Verification items for the finished model (mm, model axes). Coordinates: 2 decimals unless noted, no trailing zeros. Write each loop counter-clockwise with the first axis right and the second up, starting at its lowest first coordinate (ties: lowest second). Pieces come first, ordered by that corner, then holes. Notation, with made-up numbers: (53.5, 11.5) -> (101.5, 11.5) arc R23 ccw to (101.5, 33.5) -> close; hole circle Ø4 at (50.25, 81). An arc over 180 degrees is marked (long way). Answer in a Markdown table with one row per item.
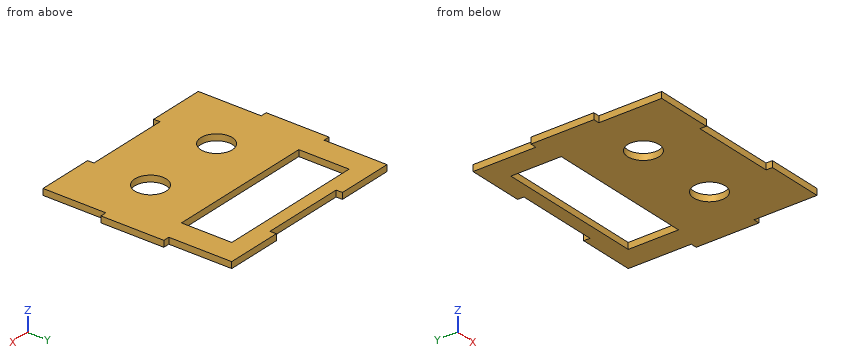
```python
from build123d import *

# Parameters (mm, degrees)
ESQUISSE1_W             = 100
ESQUISSE1_H             = 90
ESQUISSE1_R             = 7.5
ESQUISSE1_W_2           = 71
ESQUISSE1_H_2           = 24
BOSS_EXTRU_1_DEPTH      = 3
ENL_V_MAT_EXTRU_1_REACH = 90.04
ESQUISSE2_W             = 40
ESQUISSE2_H             = 3
ESQUISSE2_W_2           = 3
ESQUISSE2_H_2           = 30


with BuildPart() as part:
    # Esquisse1 → Boss.-Extru.1 (new body)
    with BuildSketch(Plane.XY):
        with Locations((-10.038524431, -19.32304038)):
            Rectangle(ESQUISSE1_W, ESQUISSE1_H)
        with Locations((-30.038524431, -34.32304038)):
            Circle(ESQUISSE1_R, mode=Mode.SUBTRACT)
        with Locations((9.961475569, -34.32304038)):
            Circle(ESQUISSE1_R, mode=Mode.SUBTRACT)
        with Locations((-10.038524431, 4.660332542)):
            Rectangle(ESQUISSE1_W_2, ESQUISSE1_H_2, mode=Mode.SUBTRACT)
    extrude(amount=BOSS_EXTRU_1_DEPTH)

    # Esquisse2 → Enlèv. mat.-Extru.1 (cut, up to next)
    with BuildSketch(Plane.XY.offset(3), mode=Mode.PRIVATE) as enl_v_mat_extru_1_sk1:
        with Locations((-10.038524431, 24.17695962)):
            Rectangle(ESQUISSE2_W, ESQUISSE2_H)
    enl_v_mat_extru_1_tool1 = extrude(enl_v_mat_extru_1_sk1.sketch, amount=-ENL_V_MAT_EXTRU_1_REACH, mode=Mode.PRIVATE) & part.part
    # Esquisse2 → Enlèv. mat.-Extru.1 (cut, up to next)
    with BuildSketch(Plane.XY.offset(3), mode=Mode.PRIVATE) as enl_v_mat_extru_1_sk2:
        with Locations((-58.538524431, 10.67695962)):
            Rectangle(ESQUISSE2_W_2, ESQUISSE2_H_2)
    enl_v_mat_extru_1_tool2 = extrude(enl_v_mat_extru_1_sk2.sketch, amount=-ENL_V_MAT_EXTRU_1_REACH, mode=Mode.PRIVATE) & part.part
    # Esquisse2 → Enlèv. mat.-Extru.1 (cut, up to next)
    with BuildSketch(Plane.XY.offset(3), mode=Mode.PRIVATE) as enl_v_mat_extru_1_sk3:
        with Locations((-58.538524431, -49.32304038)):
            Rectangle(ESQUISSE2_W_2, ESQUISSE2_H_2)
    enl_v_mat_extru_1_tool3 = extrude(enl_v_mat_extru_1_sk3.sketch, amount=-ENL_V_MAT_EXTRU_1_REACH, mode=Mode.PRIVATE) & part.part
    # Esquisse2 → Enlèv. mat.-Extru.1 (cut, up to next)
    with BuildSketch(Plane.XY.offset(3), mode=Mode.PRIVATE) as enl_v_mat_extru_1_sk4:
        with Locations((-10.038524431, -62.82304038)):
            Rectangle(ESQUISSE2_W, ESQUISSE2_H)
    enl_v_mat_extru_1_tool4 = extrude(enl_v_mat_extru_1_sk4.sketch, amount=-ENL_V_MAT_EXTRU_1_REACH, mode=Mode.PRIVATE) & part.part
    # Esquisse2 → Enlèv. mat.-Extru.1 (cut, up to next)
    with BuildSketch(Plane.XY.offset(3), mode=Mode.PRIVATE) as enl_v_mat_extru_1_sk5:
        with Locations((38.461475569, -49.32304038)):
            Rectangle(ESQUISSE2_W_2, ESQUISSE2_H_2)
    enl_v_mat_extru_1_tool5 = extrude(enl_v_mat_extru_1_sk5.sketch, amount=-ENL_V_MAT_EXTRU_1_REACH, mode=Mode.PRIVATE) & part.part
    # Esquisse2 → Enlèv. mat.-Extru.1 (cut, up to next)
    with BuildSketch(Plane.XY.offset(3), mode=Mode.PRIVATE) as enl_v_mat_extru_1_sk6:
        with Locations((38.461475569, 10.67695962)):
            Rectangle(ESQUISSE2_W_2, ESQUISSE2_H_2)
    enl_v_mat_extru_1_tool6 = extrude(enl_v_mat_extru_1_sk6.sketch, amount=-ENL_V_MAT_EXTRU_1_REACH, mode=Mode.PRIVATE) & part.part
    add(enl_v_mat_extru_1_tool1.solids().sort_by_distance((-10.038524, 24.17696, 3))[0], mode=Mode.SUBTRACT)
    add(enl_v_mat_extru_1_tool2.solids().sort_by_distance((-58.538524, 10.67696, 3))[0], mode=Mode.SUBTRACT)
    add(enl_v_mat_extru_1_tool3.solids().sort_by_distance((-58.538524, -49.32304, 3))[0], mode=Mode.SUBTRACT)
    add(enl_v_mat_extru_1_tool4.solids().sort_by_distance((-10.038524, -62.82304, 3))[0], mode=Mode.SUBTRACT)
    add(enl_v_mat_extru_1_tool5.solids().sort_by_distance((38.461476, -49.32304, 3))[0], mode=Mode.SUBTRACT)
    add(enl_v_mat_extru_1_tool6.solids().sort_by_distance((38.461476, 10.67696, 3))[0], mode=Mode.SUBTRACT)


solid = part.part
```
1. Sectioned sample at B-B, the plane x = -19. Record the cut outline in (y, z), and give its area (3 significant figures).
Findings below:
| item | result |
|---|---|
| outline | (-61.32, 0) -> (-7.34, 0) -> (-7.34, 3) -> (-61.32, 3) -> close; (16.66, 0) -> (22.68, 0) -> (22.68, 3) -> (16.66, 3) -> close |
| area | 180 mm² |
2. Sectioned sample at D-D, the plane y = -37.5. Record the cut outline in (x, z).
Findings below:
| item | result |
|---|---|
| outline | (-57.04, 0) -> (-36.83, 0) -> (-36.83, 3) -> (-57.04, 3) -> close; (-23.24, 0) -> (3.17, 0) -> (3.17, 3) -> (-23.24, 3) -> close; (16.76, 0) -> (36.96, 0) -> (36.96, 3) -> (16.76, 3) -> close |
3. Go/stop test with flat-tipped pins: pin 1 (0.9 mm diameter, centred on x = -12.5, z = 2, fed in from +Y); pin 2 (1.5 mm diameter, centred on x = -15.5, z = 1, fed in from -Y); pin 3 (0.9 mm diameter, centred on y = -62, z = 2, fed in from -X); pin 4 (10 mm diameter, centred on x = -6.5, y = -20, fed in from -Z). Record where each tip stops, or that it passes through.
Findings below:
| item | result |
|---|---|
| pin 1 | stops at y = 22.68 |
| pin 2 | stops at y = -61.32 |
| pin 3 | stops at x = -57.04 |
| pin 4 | stops at z = 0 |
4. Sectioned sample at C-C, the plane z = 2.35. Record the cut outline in (x, y).
Findings below:
| item | result |
|---|---|
| outline | (-60.04, -34.32) -> (-57.04, -34.32) -> (-57.04, -64.32) -> (-30.04, -64.32) -> (-30.04, -61.32) -> (9.96, -61.32) -> (9.96, -64.32) -> (36.96, -64.32) -> (36.96, -34.32) -> (39.96, -34.32) -> (39.96, -4.32) -> (36.96, -4.32) -> (36.96, 25.68) -> (9.96, 25.68) -> (9.96, 22.68) -> (-30.04, 22.68) -> (-30.04, 25.68) -> (-57.04, 25.68) -> (-57.04, -4.32) -> (-60.04, -4.32) -> close; hole (-45.54, -7.34) -> (25.46, -7.34) -> (25.46, 16.66) -> (-45.54, 16.66) -> close; hole circle Ø15 at (-30.04, -34.32); hole circle Ø15 at (9.96, -34.32) |
5. Sectioned sample at A-A, the plane y = 11.5. Record the cut outline in (x, z).
Findings below:
| item | result |
|---|---|
| outline | (-57.04, 0) -> (-45.54, 0) -> (-45.54, 3) -> (-57.04, 3) -> close; (25.46, 0) -> (36.96, 0) -> (36.96, 3) -> (25.46, 3) -> close |
6. Material ranges on probe 1 along Y at (x, z) = (-39.5, 0.4); probe 2 along Y at (x, z) = (-2.5, 1.5); probe 3 along X at (y, z) = (-40.5, 2.15), recorded low to high. Write a range as from..to.
Findings below:
| item | result |
|---|---|
| probe 1 | y = -64.32..-7.34, 16.66..25.68 |
| probe 2 | y = -61.32..-7.34, 16.66..22.68 |
| probe 3 | x = -57.04..-34.29, -25.78..5.71, 14.22..36.96 |
